Check sheet for the modelled part. Datum: model origin and axes. Units: mm. Face numbers are marked on the shaded views. A direction names the side the tool comes from. Round coordinates to 2 decimals unless told otherwise and drop trailing zeros. Write each loop counter-clockwise with the first axis right and the second up, starting at its lowest first coordinate (ties: lowest second). Pieces come first, ordered by that corner, then holes. Notation, with made-up numbers: (87, 52.25) -> (140, 52.25) arc R17 cw to (140, 60.25) -> close; hole circle Ø1 at (75.5, 10.25). An arc over 180 degrees is marked (long way). One line per item, written item: value. Start each with the question number.
```python
from build123d import *

# Parameters (mm, degrees)
F0_W      = 16
F0_H      = 16
F1_DEPTH  = 16
F2_R      = 7
F3_DEPTH  = 16
F4_R      = 4
F5_DEPTH  = 34
F6_R      = 3
F7_DEPTH  = 18
F6_R_2    = 5
F8_DEPTH  = 28
F9_R      = 3
F10_DEPTH = 16
F9_R_2    = 7
F11_DEPTH = 10


with BuildPart() as f1:
    # F0 (on Right) → F1 (new body)
    with BuildSketch(Plane.YZ):
        with Locations((8, 8)):
            Rectangle(F0_W, F0_H)
    extrude(amount=F1_DEPTH)

    # F2 (on face) → F3 (join)
    with BuildSketch(Plane.XY.offset(16)):
        with Locations((8, 8)):
            Circle(F2_R)
    extrude(amount=F3_DEPTH)

    # F4 (on face) → F5 (cut)
    with BuildSketch(Plane.XY.offset(32)):
        with Locations((8, 8)):
            Circle(F4_R)
    extrude(amount=-F5_DEPTH, mode=Mode.SUBTRACT)

    # F6 (on face) → F7 (cut)
    with BuildSketch(Plane.YZ.offset(16)):
        with Locations((8, 8)):
            Circle(F6_R)
    extrude(amount=-F7_DEPTH, mode=Mode.SUBTRACT)

    # F6 (on face) → F8 (join)
    with BuildSketch(Plane.YZ.offset(16)):
        with Locations((8, 8)):
            Circle(F6_R_2)
        with Locations((8, 8)):
            Circle(F6_R, mode=Mode.SUBTRACT)
    extrude(amount=F8_DEPTH)

    # F9 (on face) → F10 (join)
    with BuildSketch(Plane(origin=(0, 16, 0), x_dir=(-1, 0, 0), z_dir=(0, 1, 0))):
        with Locations((-8, 8)):
            Circle(F9_R)
    extrude(amount=F10_DEPTH)

    # F9 (on face) → F11 (join)
    with BuildSketch(Plane(origin=(0, 16, 0), x_dir=(-1, 0, 0), z_dir=(0, 1, 0))):
        with Locations((-8, 8)):
            Circle(F9_R_2)
        with Locations((-8, 8)):
            Circle(F9_R, mode=Mode.SUBTRACT)
    extrude(amount=F11_DEPTH)


solid = f1.part
```
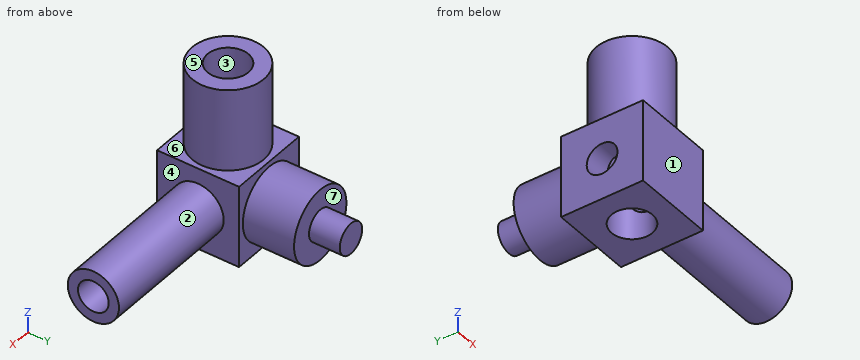
1. Material ranges on probe 1 along Y at (x, z) = (2, 8); probe 2 along Y at (x, z) = (8, 14); probe 3 along Z at (x, y) = (12.15, 8), recorded low to high.
2. Release check for a two-part mould opening along Y. For the marked faces 1, 2 and 3 record: +Y half, -Y half, draft (parallel to the pull), parting line (faces both ways), or undercut.
3. Cross-section at D-D (z = 29.5). Record the cut outline in (x, y), plus the area to 3 significant figures.
4. Cross-section at B-B (y = 8). Record the cut outline in (x, z).
5. Cross-section at C-C (z = 8). Record the cut outline in (x, y).
6. Access from +Z, -Z, +X, -X, +Y, -Y to the whole of each face (thin tool, end or side, straight path). Record for the marked faces 4, 5, 6 and 7.
7. Depth check by flat-ended pin: pin 1 Ø1 at (y, z) = (20, 4) entering from +X; pin 2 Ø8 at (x, y) = (7, 26.5) entering from +Z; pin 3 Ø2 at (y, z) = (19.5, 5.5) entering from -X. Enter the tip coordinate at first touch or a pass-through.
8. Cross-section at A-A (x = 8). Record the cut outline in (y, z), plus the area to 3 significant figures.
Working result:
1. probe 1: y = 0 to 5, 11 to 26
1. probe 2: y = 0 to 4, 12 to 26
1. probe 3: z = 0 to 5, 11 to 32
2. face 1: -Y half
2. face 2: parting line
2. face 3: undercut
3. outline: circle Ø14 at (8, 8); hole circle Ø8 at (8, 8)
3. area: 104 mm^2
4. outline: (0, 0) -> (4, 0) -> (4, 5) -> (0, 5) -> close; (0, 11) -> (4, 11) -> (4, 32) -> (1, 32) -> (1, 16) -> (0, 16) -> close; (12, 0) -> (16, 0) -> (16, 3) -> (44, 3) -> (44, 5) -> (12, 5) -> close; (12, 11) -> (44, 11) -> (44, 13) -> (16, 13) -> (16, 16) -> (15, 16) -> (15, 32) -> (12, 32) -> close
5. outline: (0, 0) -> (16, 0) -> (16, 3) -> (44, 3) -> (44, 5) -> (10.65, 5) arc R4 cw to (5.35, 5) -> (0, 5) -> close; (0, 11) -> (5.35, 11) arc R4 cw to (10.65, 11) -> (44, 11) -> (44, 13) -> (16, 13) -> (16, 16) -> (15, 16) -> (15, 26) -> (11, 26) -> (11, 32) -> (5, 32) -> (5, 26) -> (1, 26) -> (1, 16) -> (0, 16) -> close
6. face 4: +X
6. face 5: +Z, +X, -X, +Y, -Y
6. face 6: +Z
6. face 7: +Y
7. pin 1: stops at x = 14.06
7. pin 2: stops at z = 15
7. pin 3: stops at x = 1.16
8. outline: (0, 0) -> (4, 0) -> (4, 32) -> (1, 32) -> (1, 16) -> (0, 16) -> close; (12, 0) -> (16, 0) -> (16, 1) -> (26, 1) -> (26, 5) -> (32, 5) -> (32, 11) -> (26, 11) -> (26, 15) -> (16, 15) -> (16, 16) -> (15, 16) -> (15, 32) -> (12, 32) -> close
8. area: 400 mm^2
